```python
from build123d import *

# Parameters (mm, degrees)
SKETCH2_R           = 12.7
BOSS_EXTRUDE1_DEPTH = 52.5
CUT_EXTRUDE1_REACH  = 142.64
SKETCH3_R           = 3
SKETCH4_R           = 8.5
CUT_EXTRUDE2_DEPTH  = 1.275
SKETCH5_R           = 7.5
CUT_EXTRUDE3_DEPTH  = 5


with BuildPart() as part:
    # Sketch2 → Boss-Extrude1 (new, symmetric)
    with BuildSketch(Plane.XY):
        with Locations((-80, 0)):
            Circle(SKETCH2_R)
    extrude(amount=BOSS_EXTRUDE1_DEPTH, both=True)

    # Sketch3 → Cut-Extrude1 (cut, up to next)
    with BuildSketch(Plane(origin=(0, 0, -52.5), x_dir=(-1, 0, 0), z_dir=(0, 0, -1)), mode=Mode.PRIVATE) as cut_extrude1_sk1:
        with Locations((80, 0)):
            Circle(SKETCH3_R)
    cut_extrude1_tool1 = extrude(cut_extrude1_sk1.sketch, amount=-CUT_EXTRUDE1_REACH, mode=Mode.PRIVATE) & part.part
    add(cut_extrude1_tool1.solids().sort_by_distance((-80, 0, -52.5))[0], mode=Mode.SUBTRACT)

    # Sketch4 → Cut-Extrude2 (cut)
    with BuildSketch(Plane(origin=(0, 0, -52.5), x_dir=(-1, 0, 0), z_dir=(0, 0, -1))):
        with Locations((80, 0)):
            Circle(SKETCH4_R)
    extrude(amount=-CUT_EXTRUDE2_DEPTH, mode=Mode.SUBTRACT)

    # Sketch5 → Cut-Extrude3 (cut)
    with BuildSketch(Plane(origin=(0, 0, -52.5), x_dir=(-1, 0, 0), z_dir=(0, 0, -1))):
        with Locations((80, 0)):
            Circle(SKETCH5_R)
    extrude(amount=-CUT_EXTRUDE3_DEPTH, mode=Mode.SUBTRACT)


solid = part.part
```
Build history of the part. All positions in model axes, mm. A direction names the side the tool comes from. Coordinates: 2 decimals unless noted, no trailing zeros. Order: outer loops, then holes, each group sorted by start corner. A loop starts at its lowest first (then second) coordinate and runs counter-clockwise, first axis right, second up.
Item 1: Drill centre lines: L1, parallel to Y at x = -80, z = -48.7; L2, parallel to Y at x = -80, z = 13.5; L3, parallel to Z at x = -73.75, y = 1.5. Where is each one in solid material? Low to high.
Filled in:
L1: y = -12.7 to -7.5, 7.5 to 12.7
L2: y = -12.7 to -3, 3 to 12.7
L3: z = -47.5 to 52.5
Item 2: Saw through at D-D on y = 4.5. List the corners of the cut face in (x, z) (3 decimals).
Filled in:
outline: (-91.876, -52.5) - (-87.211, -52.5) - (-87.211, -51.225) - (-86, -51.225) - (-86, -47.5) - (-74, -47.5) - (-74, -51.225) - (-72.789, -51.225) - (-72.789, -52.5) - (-68.124, -52.5) - (-68.124, 52.5) - (-91.876, 52.5) - close
Item 3: Saw through at C-C on z = 27. List the corners of the cut face in (x, y).
Filled in:
outline: circle Ø25.4 at (-80, 0); hole circle Ø6 at (-80, 0)
Item 4: Tool access for faces 5 (the flat face through (-77, -3, 52.5)), 6 (the flat face through (-79.9, -3.2, -47.5)): list every direction of +Z, -Z, +X, -X, +Y, -Y with a clear straight run to the whole face (end or side of a thin tool).
Filled in:
face 5: +Z, +X, -X, +Y, -Y
face 6: -Z
Item 5: Drop flat-ended pins along their axis: pin 1 Ø2 at (x, z) = (-70, 5) entering from +Y; pin 2 Ø3 at (y, z) = (-2, 40) entering from +X; pin 3 Ø1 at (x, y) = (-81, -6.5) entering from -Z. Give the stop position or say it passes through.
Filled in:
pin 1: stops at y = 8.96
pin 2: stops at x = -67.31
pin 3: stops at z = -47.5
Item 6: Saw through at B-B on y = 0. List the corners of the cut face in (x, z) (3 decimals).
Filled in:
outline: (-92.7, -52.5) - (-88.5, -52.5) - (-88.5, -51.225) - (-87.5, -51.225) - (-87.5, -47.5) - (-83, -47.5) - (-83, 52.5) - (-92.7, 52.5) - close; (-77, -47.5) - (-72.5, -47.5) - (-72.5, -51.225) - (-71.5, -51.225) - (-71.5, -52.5) - (-67.3, -52.5) - (-67.3, 52.5) - (-77, 52.5) - close
Item 7: Saw through at A-A on x = -80. List the corners of the cut face in (y, z) (3 decimals), then the cut area to 3 significant figures.
Filled in:
outline: (-12.7, -52.5) - (-8.5, -52.5) - (-8.5, -51.225) - (-7.5, -51.225) - (-7.5, -47.5) - (-3, -47.5) - (-3, 52.5) - (-12.7, 52.5) - close; (3, -47.5) - (7.5, -47.5) - (7.5, -51.225) - (8.5, -51.225) - (8.5, -52.5) - (12.7, -52.5) - (12.7, 52.5) - (3, 52.5) - close
area: 1,990 mm2
Item 8: Mould opens along X. For faces 1 (the cylindrical face through (-71.51, 0.37, -51.87)), 2 (the flat face through (-77.4, -8.3, -52.5)), 3 (the cylindrical face through (-77, 0, 2)), 4 (the cylindrical face through (-92.688, 0.558, 0.735)) say: released by +X, released by -X, zero draft, split by the parting line, or undercut.
Filled in:
face 1: undercut
face 2: zero draft
face 3: undercut
face 4: split by the parting line
